```python
from build123d import *

# Parameters (mm, degrees)
SKETCH1_R                    = 2.65
SKETCH1_R_2                  = 13.5
BOSS_EXTRUDE1_DEPTH          = 6.35
M2_5X0_45_TAPPED_HOLE1_D     = 2.05
M2_5X0_45_TAPPED_HOLE2_D     = 2.05
M2_5X0_45_TAPPED_HOLE2_DEPTH = 6.35
M2_5X0_45_TAPPED_HOLE2_TIP   = 0.615882135


with BuildPart() as part:
    # Sketch1 → Boss-Extrude1 (new body)
    with BuildSketch(Plane(origin=(0, 0, 0), x_dir=(0, 0, -1), z_dir=(1, 0, 0))):
        with BuildLine():
            Line((-50, 29.5), (0, 29.5))
            Line((0, 29.5), (0, -29.5))
            Line((0, -29.5), (-50, -29.5))
            ThreePointArc((-50, -29.5), (-79.5, 0), (-50, 29.5))
        make_face()
        with Locations((-60.75, -18.619546181)):
            Circle(SKETCH1_R, mode=Mode.SUBTRACT)
        with Locations((-28.5, 0)):
            Circle(SKETCH1_R, mode=Mode.SUBTRACT)
        with Locations((-60.75, 18.619546181)):
            Circle(SKETCH1_R, mode=Mode.SUBTRACT)
        with Locations((-50, 0)):
            Circle(SKETCH1_R_2, mode=Mode.SUBTRACT)
    extrude(amount=BOSS_EXTRUDE1_DEPTH)

    # M2.5x0.45 Tapped Hole1 (through all)
    with Locations(Plane(origin=(6.35, 0, 0), x_dir=(0, 0, -1), z_dir=(1, 0, 0))):
        with Locations((-50, -23.015), (-50, 23.015)):
            Hole(M2_5X0_45_TAPPED_HOLE1_D / 2)

    # M2.5x0.45 Tapped Hole2
    with Locations(Plane(origin=(0, 0, 0), x_dir=(-1, 0, 0), z_dir=(0, 0, -1))):
        with Locations((-3.175, 0), (-3.175, 12.75), (-3.175, 25.5), (-3.175, -12.75), (-3.175, -25.5)):
            Hole(M2_5X0_45_TAPPED_HOLE2_D / 2, depth=M2_5X0_45_TAPPED_HOLE2_DEPTH)
            with Locations((0, 0, -(M2_5X0_45_TAPPED_HOLE2_DEPTH + M2_5X0_45_TAPPED_HOLE2_TIP / 2))):  # 118° drill point
                Cone(0, M2_5X0_45_TAPPED_HOLE2_D / 2, M2_5X0_45_TAPPED_HOLE2_TIP, mode=Mode.SUBTRACT)


solid = part.part
```
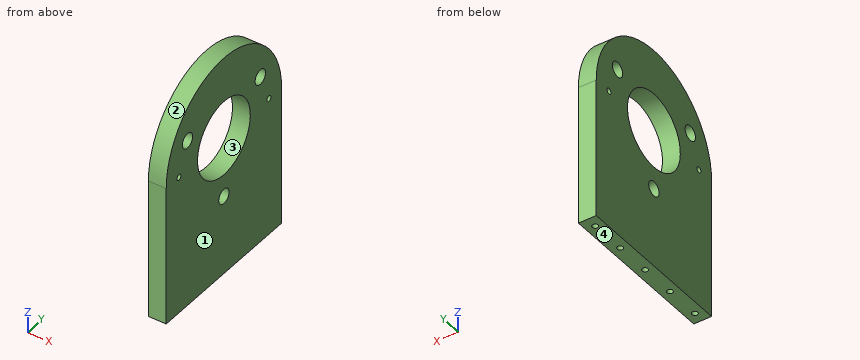
Part model, mm, in its own coordinate system. Face numbers are marked on the shaded views. Give positions to 0.01 mm unless a question says otherwise; leave off trailing zeros. Order: outer loops, then holes, each group sorted by start corner. A loop starts at its lowest first (then second) coordinate and runs counter-clockwise, first axis right, second up. Notation, with made-up numbers: (2, -9) - (48, -9) arc R22 ccw to (48, 3) - close; hole circle Ø11 at (47, 87.25). An arc over 180 degrees is marked (long way). Use one line per item in the form item = value.
Item 1: Slice it at A-A on z = 28.5. Give the cut face in (x, y), and give its area (3 significant figures).
Solution:
outline = (0, -29.5) - (6.35, -29.5) - (6.35, -2.65) - (0, -2.65) - close; (0, 2.65) - (6.35, 2.65) - (6.35, 29.5) - (0, 29.5) - close
area = 341 mm2
Item 2: Slice it at B-B on x = 5.5. Give the cut face in (y, z) (3 decimals).
Solution:
outline = (-29.5, 0) - (29.5, 0) - (29.5, 50) arc R29.5 ccw to (-29.5, 50) - close; hole circle Ø2.05 at (-23.015, 50); hole circle Ø5.3 at (-18.62, 60.75); hole circle Ø27 at (0, 50); hole circle Ø5.3 at (0, 28.5); hole circle Ø5.3 at (18.62, 60.75); hole circle Ø2.05 at (23.015, 50)
Item 3: Probe probe 1 along Y at (x, z) = (4.5, 50); probe 2 along Y at (x, z) = (3, 28.5); probe 3 along Z at (x, y) = (1.25, -1.5). List the from-to ranges inside material, lowest first. Write a range as from..to.
Solution:
probe_1 = -29.5..-24.04, -21.99..-13.5, 13.5..21.99, 24.04..29.5
probe_2 = -29.5..-2.65, 2.65..29.5
probe_3 = 0..26.32, 30.68..36.58, 63.42..79.46
Item 4: Pin check, flat tips, straight feed: pin 1 Ø1.8 at (x, y) = (3.175, 25.5) entering from +Z; pin 2 Ø1.6 at (x, y) = (3.175, 12.75) entering from -Z; pin 3 Ø2 at (x, z) = (3, 63) entering from +Y. Stop position of each tip, or through.
Solution:
pin_1 = 66.28
pin_2 = 6.49
pin_3 = 26.95
Item 5: Slice it at D-D on z = 70. Give the cut face in (x, y), and give its area (3 significant figures).
Solution:
outline = (0, -21.69) - (6.35, -21.69) - (6.35, 21.69) - (0, 21.69) - close
area = 275 mm2
Item 6: Slice it at C-C on y = 7.5. Give the cut face in (x, z), and give its area (3 significant figures).
Solution:
outline = (0, 0) - (6.35, 0) - (6.35, 38.78) - (0, 38.78) - close; (0, 61.22) - (6.35, 61.22) - (6.35, 78.53) - (0, 78.53) - close
area = 356 mm2
Item 7: Two-plate mould, pull along Z, no slides. Class the marked faces 1, 2, 3 and 4: released by +Z, released by -Z, zero draft, split by the parting line, or undercut.
Solution:
face_1 = zero draft
face_2 = released by +Z
face_3 = undercut
face_4 = released by -Z
